Part print with two shaded views. Sizes in mm from the minimum x, y, z corner. A direction names the side the tool comes from. Coordinates: 2 decimals unless noted, no trailing zeros. Order: outer loops, then holes, each group sorted by start corner. A loop starts at its lowest first (then second) coordinate and runs counter-clockwise, first axis right, second up.
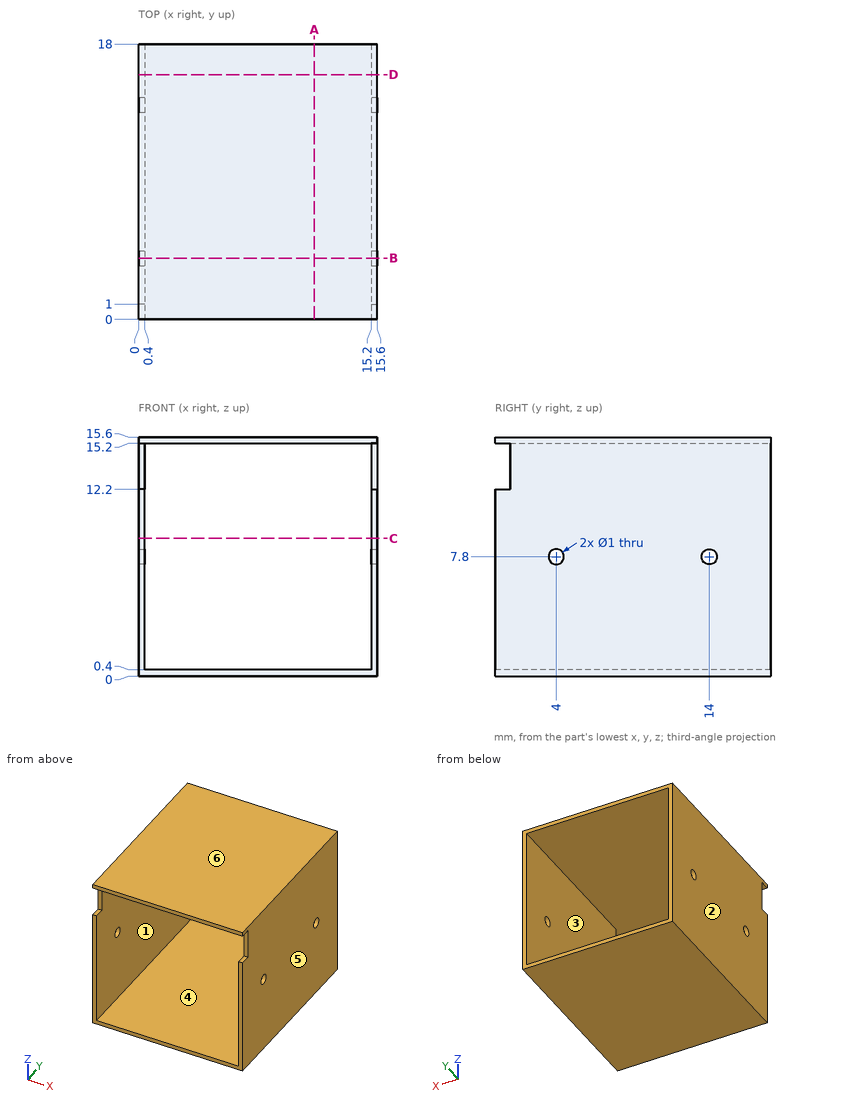
Q1. Mould opens along X. For the marked faces 3, 4, 5 and 6 say: pulls with the +X half, pulls with the -X half, needs draft (parallel to the pull), parting line crosses it, or undercut.
Results list:
face 3: undercut
face 4: undercut
face 5: pulls with the +X half
face 6: needs draft
Q2. Wall check: line 1 along Y through (x, z) = (15.35, 7.8); line 2 along Z through (x, y) = (6.25, 13.5); line 3 along Z through (x, y) = (0.1, 14). Give the ranges that are in metal, low to high.
Results list:
line 1: y = 0 to 3.5, 4.5 to 13.5, 14.5 to 18
line 2: z = 0 to 0.4, 15.2 to 15.6
line 3: z = 0 to 7.3, 8.3 to 15.6
Q3. Cut at A-A on x = 11.5. Write the cut outline in (y, z), and give its area (3 significant figures).
Results list:
outline: (0, 0) - (18, 0) - (18, 0.4) - (0, 0.4) - close; (0, 15.2) - (18, 15.2) - (18, 15.6) - (0, 15.6) - close
area: 14.4 mm2
Q4. Cut at C-C on z = 9. Write the cut outline in (x, y).
Results list:
outline: (0, 0) - (0.4, 0) - (0.4, 18) - (0, 18) - close; (15.2, 0) - (15.6, 0) - (15.6, 18) - (15.2, 18) - close
Q5. Which spindle directions (+Z, -Z, +X, -X, +Y, -Y) get a long thin tool onto all of the face, cutting with end or side? Do the marked faces 1 and 2. Say none if no direction does.
Results list:
face 1: +Y, -Y
face 2: +Z, -Z, -X, +Y, -Y
Q6. Cut at D-D on y = 16. Write the cut outline in (x, z).
Results list:
outline: (0, 0) - (15.6, 0) - (15.6, 15.6) - (0, 15.6) - close; hole (0.4, 0.4) - (15.2, 0.4) - (15.2, 15.2) - (0.4, 15.2) - close
Q7. Cut at B-B on y = 4. Write the cut outline in (x, z), and give its area (3 significant figures).
Results list:
outline: (0, 0) - (15.6, 0) - (15.6, 7.3) - (15.2, 7.3) - (15.2, 0.4) - (0.4, 0.4) - (0.4, 7.3) - (0, 7.3) - close; (0, 8.3) - (0.4, 8.3) - (0.4, 15.2) - (15.2, 15.2) - (15.2, 8.3) - (15.6, 8.3) - (15.6, 15.6) - (0, 15.6) - close
area: 23.5 mm2
